Build history of the part. All positions in model axes, mm. Face numbers are marked on the shaded views. Coordinates: 2 decimals unless noted, no trailing zeros. Order: outer loops, then holes, each group sorted by start corner. A loop starts at its lowest first (then second) coordinate and runs counter-clockwise, first axis right, second up. Notation, with made-up numbers: M -22.75,79.5 L -0.75,79.5 A19 cw -0.75,98.5 Z; hole C 44,-19 d8. An arc over 180 degrees is marked long. Write item = value, one per line. Start each with the question number.
Q1. Band-saw the part on B-B on x = 32. Write the cut outline in (y, z), plus the area to 3 significant figures.
Q2. Drill centre lines: probe 1 along Z at (x, y) = (0, 18.5); probe 2 along X at (y, z) = (35.5, 1.7); probe 3 along X at (y, z) = (25, 1.9). Where is each one in solid material? Low to high.
Q3. Band-saw the part on C-C on z = 0.85. Write the cut outline in (x, y).
Q4. Pin check, flat tips, straight feed: P1, Ø1, axis at x = -3.5, y = 21.5, coming from the -Z side; P2, Ø21, axis at x = 0, y = 31.5, coming from the -Z side; P3, Ø8, axis at x = 29.5, y = 29, coming from the +Z side. Stop position of each tip, or through.
Q5. Band-saw the part on D-D on y = 60.5. Write the cut outline in (x, z), plus the area to 3 significant figures.
Q6. Pull direction X, two halves, no side cores. Call the marked faces 1 and 2: released by +X, released by -X, zero draft, split by the parting line, or undercut.
```python
from build123d import *

# Parameters (mm, degrees)
F1_DEPTH = 4
F2_DEPTH = 2
F3_START = 2
F3_DEPTH = 2
F4_SIZE  = 1.99999


# Not quite as in the source:
# - a fillet or chamfer is up to 0.001 mm smaller than in the source, because OpenCascade refuses the exact size


with BuildPart() as f1:
    # F0 (on Top) → F1 (new body)
    with BuildSketch(Plane.XY):
        Polygon((32.7846783229, 14.824549064), (4.8026783229, 63.2907947614), (-23.1793216771, 14.824549064), align=None)
        Polygon((-19.715220062, 16.824549064), (4.8026783229, 59.2907947614), (29.3205767077, 16.824549064), align=None, mode=Mode.SUBTRACT)
    extrude(amount=F1_DEPTH)

    # F0 (on Top) → F2 (join)
    with BuildSketch(Plane.XY):
        Polygon((37.1148053418, 12.324549064), (4.8026783229, 68.2907947614), (-27.509448696, 12.324549064), align=None)
        Polygon((-23.1793216771, 14.824549064), (4.8026783229, 63.2907947614), (32.7846783229, 14.824549064), align=None, mode=Mode.SUBTRACT)
    extrude(amount=F2_DEPTH)

    # F0 (on Top) → F3 (join)
    with BuildSketch(Plane.XY.offset(F3_START)):
        Polygon((29.3205767077, 16.824549064), (4.8026783229, 59.2907947614), (-19.715220062, 16.824549064), align=None)
    extrude(amount=F3_DEPTH)

    # F4 (size 2 in the source; OpenCascade refuses exactly that, so slightly less here)
    f4_edges = [f1.edges().sort_by_distance(p)[0] for p in [
        (4.802678, 16.824549, 0),
        (-7.456271, 38.057672, 0),
        (17.061628, 38.057672, 0),
    ]]
    chamfer(f4_edges, length=F4_SIZE)


solid = f1.part
```
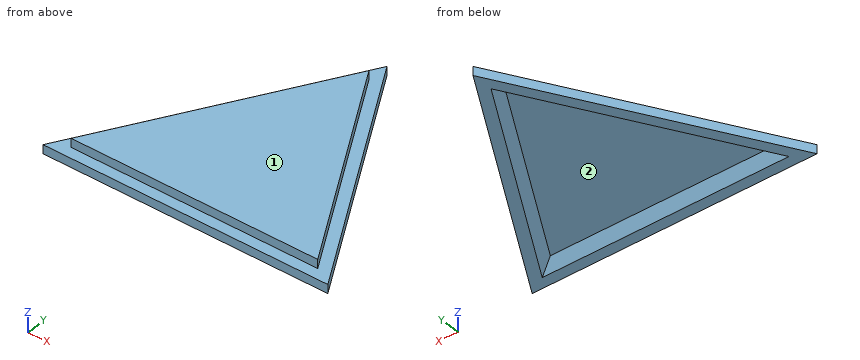
Recorded:
q1.outline = M 12.32,0 L 14.82,0 L 15.28,0.45 L 16.18,0 L 21.18,0 L 21.18,2 L 16.18,2 L 16.18,4 L 14.82,4 L 14.82,2 L 12.32,2 Z
q1.area = 20.1 mm2
q2.probe_1 = 2 to 4
q2.probe_2 = -14.13 to -9.28, 18.88 to 23.73
q2.probe_3 = -20.19 to -15.11, 24.72 to 29.8
q3.outline = M -27.51,12.32 L 37.11,12.32 L 4.8,68.29 Z; hole M -21.71,15.67 L 31.31,15.67 L 4.8,61.59 Z
q4.P1 = 2
q4.P2 = 1.24
q4.P3 = 2
q5.outline = M 0.3,0 L 3.19,0 L 4.8,1.4 L 6.41,0 L 9.3,0 L 9.3,2 L 6.41,2 L 6.41,4 L 3.19,4 L 3.19,2 L 0.3,2 Z
q5.area = 22.2 mm2
q6.face_1 = zero draft
q6.face_2 = undercut
